Source: three-view drawing plus pictorial views. Frame: mm from the lowest corner of the part. Round coordinates to 2 decimals unless told otherwise and drop trailing zeros. Order: outer loops, then holes, each group sorted by start corner. A loop starts at its lowest first (then second) coordinate and runs counter-clockwise, first axis right, second up. Notation, with made-up numbers: (-7, 9) - (39, 9) arc R6 cw to (39, 17) - close; hole circle Ø7 at (57, 66). An arc over 180 degrees is marked (long way). Use one line per item in the form item = value. Start each with the question number.
Q1. Pin query (flat end, axial travel): pin 1 Ø4 at (x, z) = (68, 28.5) entering from -Y; pin 2 Ø10 at (x, z) = (19.05, 19.05) entering from -Y; pin 3 Ø1 at (x, y) = (89.5, 1.5) entering from +Z. Return the tip coordinate at first contact, or that it passes through.
Q2. Ray query, line 1 (X direction, y = 0.75, z = 38); line 2 (X direction, y = 3.75, z = 35); line 3 (Z direction, x = 82.55, y = 4). Return the intervals inside material, ascending. Write a range as [from, to].
Q3. Cut plane D-D, the plane x = 82.55. Return the cut outline in (y, z).
Q4. Cut plane B-B, the plane y = 2. Give the number of separate pieces and of enclosed holes in the cut face, and give its area (3 significant figures).
Q5. Draft query along Z for the marked faces 1, 2, 3 and 4. Return one class per face: released by +Z, released by -Z, zero draft, split by the parting line, or undercut.
Q6. Cut plane C-C, the plane z = 21. Return the cut outline in (x, y).
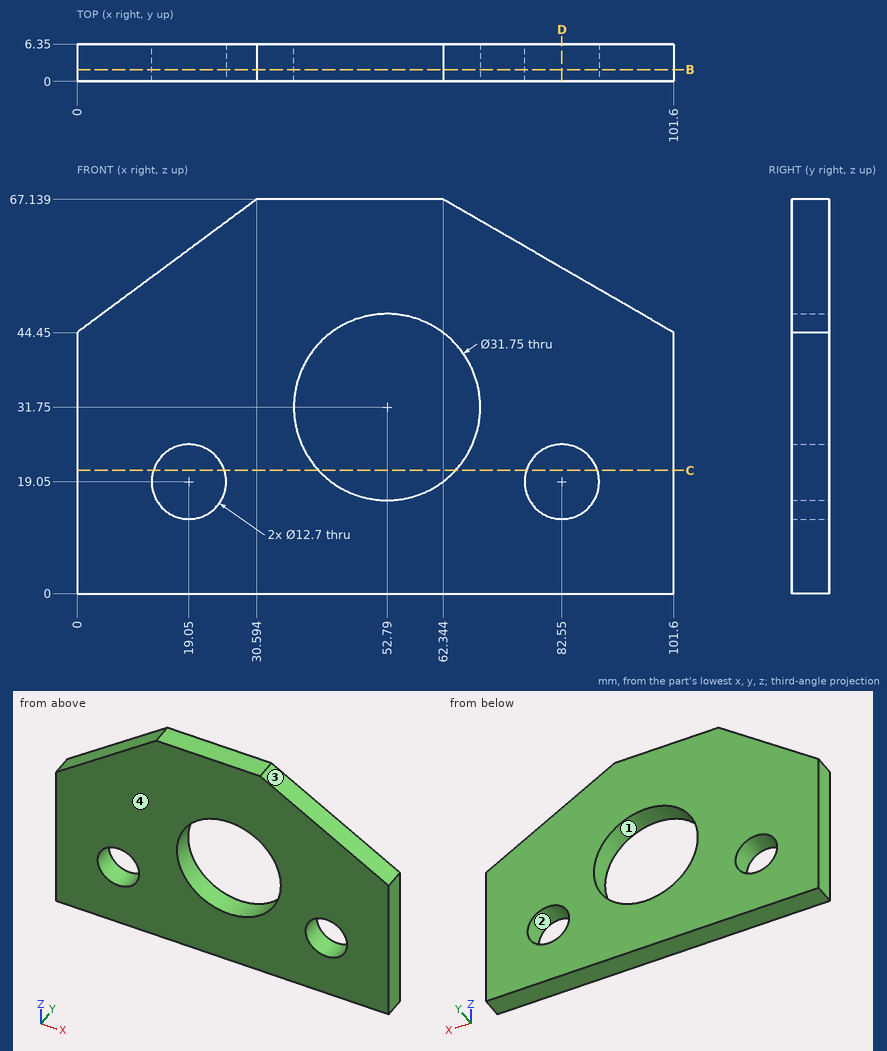
Completed:
q1.pin_1 = 0
q1.pin_2 = through
q1.pin_3 = 51.73
q2.line_1 = [0, 38.2], [67.38, 101.6]
q2.line_2 = [0, 37.25], [68.33, 101.6]
q2.line_3 = [0, 12.7], [25.4, 55.46]
q3.outline = (0, 0) - (6.35, 0) - (6.35, 12.7) - (0, 12.7) - close; (0, 25.4) - (6.35, 25.4) - (6.35, 55.46) - (0, 55.46) - close
q4.separate_pieces = 1
q4.enclosed_holes = 3
q4.area = 4,980 mm2
q5.face_1 = undercut
q5.face_2 = undercut
q5.face_3 = released by +Z
q5.face_4 = zero draft
q6.outline = (0, 0) - (13.01, 0) - (13.01, 6.35) - (0, 6.35) - close; (25.09, 0) - (41.11, 0) - (41.11, 6.35) - (25.09, 6.35) - close; (64.47, 0) - (76.51, 0) - (76.51, 6.35) - (64.47, 6.35) - close; (88.59, 0) - (101.6, 0) - (101.6, 6.35) - (88.59, 6.35) - close
